from build123d import *

# Parameters (mm, degrees)
SKETCH_R             = 80
SKETCH_R_2           = 15
SKETCH_R_3           = 1
PAD_DEPTH            = 3
SKETCH001_R          = 30
SKETCH001_R_2        = 27
PAD001_DEPTH         = 15
SKETCH002_R          = 6
PAD002_DEPTH         = 15
SKETCH004_R          = 1.6
POCKET_DEPTH         = 15.001
SKETCH003_R          = 4
POCKET001_DEPTH      = 3
SKETCH005_R          = 1
POCKET002_DEPTH      = 80.001
POCKET002_DEPTH_BACK = -80.001
POCKET003_DEPTH      = 6


with BuildPart() as part:
    # Sketch → Pad (new body)
    with BuildSketch(Plane.XY):
        Circle(SKETCH_R)
        Circle(SKETCH_R_2, mode=Mode.SUBTRACT)
        with Locations((-66.683956, 38.5)):
            Circle(SKETCH_R_3, mode=Mode.SUBTRACT)
        with Locations((66.683956, 38.5)):
            Circle(SKETCH_R_3, mode=Mode.SUBTRACT)
        with Locations((0, -77)):
            Circle(SKETCH_R_3, mode=Mode.SUBTRACT)
        with BuildLine():
            ThreePointArc((-15, 45), (0, 30), (15, 45))
            Line((15, 45), (15, 60))
            ThreePointArc((15, 60), (0, 75), (-15, 60))
            Line((-15, 45), (-15, 60))
        make_face(mode=Mode.SUBTRACT)
        with BuildLine():
            ThreePointArc((-31.471143, -35.490381), (-25.980762, -15), (-46.471143, -9.509619))
            Line((-46.471143, -9.509619), (-59.461524, -17.009619))
            ThreePointArc((-59.461524, -17.009619), (-64.951905, -37.5), (-44.461524, -42.990381))
            Line((-31.471143, -35.490381), (-44.461524, -42.990381))
        make_face(mode=Mode.SUBTRACT)
        with BuildLine():
            ThreePointArc((46.471143, -9.509619), (25.980762, -15), (31.471143, -35.490381))
            Line((31.471143, -35.490381), (44.461524, -42.990381))
            ThreePointArc((44.461524, -42.990381), (64.951905, -37.5), (59.461524, -17.009619))
            Line((46.471143, -9.509619), (59.461524, -17.009619))
        make_face(mode=Mode.SUBTRACT)
    extrude(amount=PAD_DEPTH)

    # Sketch001 → Pad001 (join)
    with BuildSketch(Plane.XY):
        Circle(SKETCH001_R)
        Circle(SKETCH001_R_2, mode=Mode.SUBTRACT)
    extrude(amount=PAD001_DEPTH)

    # Sketch002 → Pad002 (join)
    with BuildSketch(Plane.XY):
        with Locations((-20.78461, 12)):
            Circle(SKETCH002_R)
        with Locations((0, -24)):
            Circle(SKETCH002_R)
        with Locations((20.78461, 12)):
            Circle(SKETCH002_R)
    extrude(amount=PAD002_DEPTH)

    # Sketch004 → Pocket (cut, through all)
    with BuildSketch(Plane.XY):
        with Locations((-20.78461, 12)):
            Circle(SKETCH004_R)
        with Locations((20.78461, 12)):
            Circle(SKETCH004_R)
        with Locations((0, -24)):
            Circle(SKETCH004_R)
    extrude(amount=POCKET_DEPTH, mode=Mode.SUBTRACT)

    # Sketch003 → Pocket001 (cut)
    with BuildSketch(Plane.XY):
        with Locations((-20.78461, 12)):
            Circle(SKETCH003_R)
        with Locations((20.78461, 12)):
            Circle(SKETCH003_R)
        with Locations((0, -24)):
            Circle(SKETCH003_R)
    extrude(amount=POCKET001_DEPTH, mode=Mode.SUBTRACT)

    # Sketch005 → Pocket002 (cut, two sides)
    with BuildSketch(Plane.YZ) as pocket002_sk:
        with Locations((-28, 10)):
            Circle(SKETCH005_R)
    extrude(amount=-POCKET002_DEPTH, mode=Mode.SUBTRACT)
    extrude(pocket002_sk.sketch, amount=-POCKET002_DEPTH_BACK, mode=Mode.SUBTRACT)

    # Sketch006 → Pocket003 (cut)
    with BuildSketch(Plane.XY):
        Polygon((-17.90961, 10.340118), (-17.90961, 13.659882), (-20.78461, 15.319764), (-23.65961, 13.659882), (-23.65961, 10.340118), (-20.78461, 8.680236), align=None)
        Polygon((20.78461, 8.680236), (23.65961, 10.340118), (23.65961, 13.659882), (20.78461, 15.319764), (17.90961, 13.659882), (17.90961, 10.340118), align=None)
        Polygon((2.875, -25.659882), (2.875, -22.340118), (0, -20.680236), (-2.875, -22.340118), (-2.875, -25.659882), (0, -27.319764), align=None)
    extrude(amount=POCKET003_DEPTH, mode=Mode.SUBTRACT)


solid = part.part
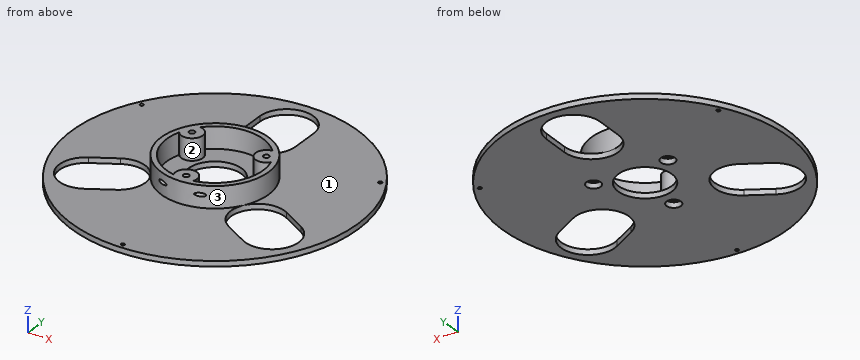
Source: CAD feature listing. Evaluate the final solid. Frame: model axes, mm. Face numbers are marked on the shaded views. Coordinates: 2 decimals unless noted, no trailing zeros. Order: outer loops, then holes, each group sorted by start corner. A loop starts at its lowest first (then second) coordinate and runs counter-clockwise, first axis right, second up. Notation, with made-up numbers: M 28,-14 L 73,-14 A28 cw 73,7 Z; hole C 4.5,81.25 d5. An arc over 180 degrees is marked long. Write each question's results on one line, items separated by ' | '. Start each with the question number.
Item 1: Line query: probe 1 along Y at (x, z) = (0, 2.05); probe 2 along Y at (x, z) = (-21, 12); probe 3 along X at (y, z) = (-6.5, 6.75). Output: solid intervals per line, ascending.
Item 2: Cut plane C-C (y = 23.5). Return loops of the section in (x, z), and give its area (3 significant figures).
Item 3: Cut plane A-A (y = 0). Return loops of the section in (x, z).
Item 4: Draft query along X for the marked faces 1, 2 and 3. Return one class per face: pulls with the +X half, pulls with the -X half, needs draft (parallel to the pull), parting line crosses it, or undercut.
Item 5: First-contact query: pin 1 Ø0.9 at (y, z) = (-25, 5) entering from +X; pin 2 Ø0.9 at (y, z) = (-25, 4) entering from -X; pin 3 Ø7 at (x, y) = (-20.78, 12) entering from -Z. Flat tips, straight axial feed; report the tip coordinate or a pass-through.
Item 6: Cut plane B-B (x = 8). Return loops of the section in (y, z).
Checked values:
1) probe 1: y = -80 to -78, -76 to -28, -20 to -15, 15 to 30, 75 to 80 | probe 2: y = -21.42 to -16.97, 6 to 10.41, 13.59 to 21.42 | probe 3: x = -29.29 to -26.21, 26.21 to 29.29
2) outline: M -76.47,0 L 76.47,0 L 76.47,3 L 18.65,3 L 18.65,15 L 13.29,15 L 13.29,3 L -13.29,3 L -13.29,15 L -18.65,15 L -18.65,3 L -76.47,3 Z | area: 587 mm2
3) outline: M -80,0 L -15,0 L -15,3 L -27,3 L -27,15 L -30,15 L -30,3 L -80,3 Z; M 15,0 L 80,0 L 80,3 L 30,3 L 30,15 L 27,15 L 27,3 L 15,3 Z
4) face 1: needs draft | face 2: undercut | face 3: parting line crosses it
5) pin 1: stops at x = 17.24 | pin 2: stops at x = -17.24 | pin 3: stops at z = 3
6) outline: M -79.6,0 L -12.69,0 L -12.69,3 L -25.79,3 L -25.79,15 L -28.91,15 L -28.91,10.41 A1 cw long -28.91,9.59 L -28.91,3 L -79.6,3 Z; M 12.69,0 L 32.31,0 L 32.31,3 L 28.91,3 L 28.91,15 L 25.79,15 L 25.79,3 L 12.69,3 Z; M 72.69,0 L 79.6,0 L 79.6,3 L 72.69,3 Z
